from build123d import *

# Parameters (mm, degrees)
SKETCH1_W            = 12.7
SKETCH1_H            = 12.7
SKETCH1_R            = 1.25
BOSS_EXTRUDE1_DEPTH  = 3.175
SKETCH2_R            = 0.75
BOSS_EXTRUDE2_DEPTH  = 1.5
SKETCH3_R            = 0.75
CUT_EXTRUDE1_DEPTH   = 1.5
SKETCH4_W            = 12.7
SKETCH4_H            = 1
CUT_EXTRUDE2_DEPTH   = 1.75
SKETCH5_W            = 7
SKETCH5_H            = 1
CUT_EXTRUDE3_DEPTH   = 0.75
FILLET1_R            = 0.25
FILLET2_R            = 0.5
FILLET1_OF_MIRROR3_R = 0.25


with BuildPart() as part:
    # Sketch1 → Boss-Extrude1 (new body)
    with BuildSketch(Plane(origin=(0, 0, 0), x_dir=(1, 0, 0), z_dir=(0, 1, 0))):
        with Locations((-6.35, 6.35)):
            Rectangle(SKETCH1_W, SKETCH1_H)
        with Locations((-2.5, 6.35)):
            Circle(SKETCH1_R, mode=Mode.SUBTRACT)
        with Locations((-10.2, 6.35)):
            Circle(SKETCH1_R, mode=Mode.SUBTRACT)
    extrude(amount=BOSS_EXTRUDE1_DEPTH)

    # Sketch2 → Boss-Extrude2 (add)
    with BuildSketch(Plane(origin=(0, 3.175, 0), x_dir=(1, 0, 0), z_dir=(0, 1, 0))):
        with Locations((-11.2, 11.2)):
            Circle(SKETCH2_R)
    boss_extrude2 = extrude(amount=BOSS_EXTRUDE2_DEPTH)

    # Sketch3 → Cut-Extrude1 (cut)
    with BuildSketch(Plane(origin=(0, 3.175, 0), x_dir=(1, 0, 0), z_dir=(0, 1, 0))):
        with Locations((-1.5, 11.2)):
            Circle(SKETCH3_R)
    cut_extrude1 = extrude(amount=-CUT_EXTRUDE1_DEPTH, mode=Mode.SUBTRACT)

    # Mirror1: Boss-Extrude2 across plane
    add(boss_extrude2.mirror(Plane(origin=(-6.35, 0, -6.35), x_dir=(-0.707106781, 0, 0.707106781), z_dir=(-0.707106781, 0, -0.707106781))))

    # Mirror2: Cut-Extrude1 across plane
    add(cut_extrude1.mirror(Plane(origin=(0, 0, 0), x_dir=(0.707106781, 0, 0.707106781), z_dir=(-0.707106781, 0, 0.707106781))), mode=Mode.SUBTRACT)

    # Sketch4 → Cut-Extrude2 (cut)
    with BuildSketch(Plane(origin=(0, 3.175, 0), x_dir=(1, 0, 0), z_dir=(0, 1, 0))):
        with Locations((-6.35, 9.2)):
            Rectangle(SKETCH4_W, SKETCH4_H)
    cut_extrude2 = extrude(amount=-CUT_EXTRUDE2_DEPTH, mode=Mode.SUBTRACT)

    # Sketch5 → Cut-Extrude3 (cut)
    with BuildSketch(Plane(origin=(0, 1.425, 0), x_dir=(1, 0, 0), z_dir=(0, 1, 0))):
        with Locations((-6.35, 9.2)):
            Rectangle(SKETCH5_W, SKETCH5_H)
    cut_extrude3 = extrude(amount=-CUT_EXTRUDE3_DEPTH, mode=Mode.SUBTRACT)

    # Fillet1
    fillet1_edges = [part.edges().sort_by_distance(p)[0] for p in [
        (-9.85, 0.675, -9.2),
        (-2.85, 0.675, -9.2),
        (-9.85, 1.425, -9.2),
        (-2.85, 1.425, -9.2),
    ]]
    fillet(fillet1_edges, radius=FILLET1_R)

    # Fillet2
    fillet2_edges = [part.edges().sort_by_distance(p)[0] for p in [
        (0, 1.5875, 0),
        (-12.7, 1.5875, 0),
        (-12.7, 1.5875, -12.7),
        (0, 1.5875, -12.7),
    ]]
    fillet(fillet2_edges, radius=FILLET2_R)

    # Mirror3: Cut-Extrude2, Cut-Extrude3 across plane
    add(cut_extrude2.mirror(Plane(origin=(0, 0, -6.35), x_dir=(1, 0, 0), z_dir=(0, 0, -1))), mode=Mode.SUBTRACT)
    add(cut_extrude3.mirror(Plane(origin=(0, 0, -6.35), x_dir=(1, 0, 0), z_dir=(0, 0, -1))), mode=Mode.SUBTRACT)

    # Fillet1 of Mirror3
    fillet1_of_mirror3_edges = [part.edges().sort_by_distance(p)[0] for p in [
        (-9.85, 0.675, -3.5),
        (-2.85, 0.675, -3.5),
        (-9.85, 1.425, -3.5),
        (-2.85, 1.425, -3.5),
    ]]
    fillet(fillet1_of_mirror3_edges, radius=FILLET1_OF_MIRROR3_R)


solid = part.part
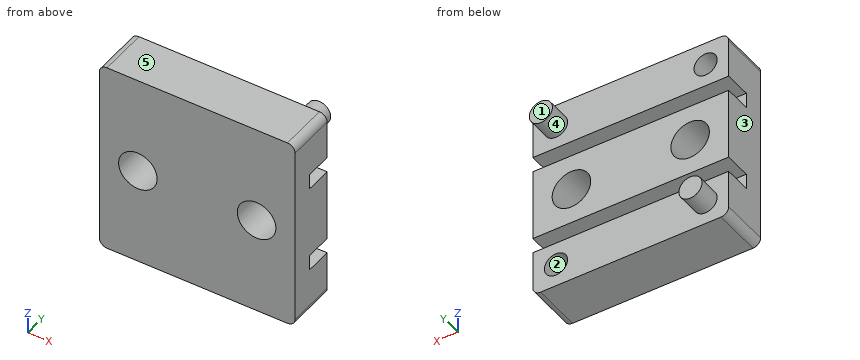
Read the model definition and answer for the solid it produces. Units are mm, in the model's axes. Face numbers are marked on the shaded views. A direction names the side the tool comes from. Give positions to 0.01 mm unless a question says otherwise; leave off trailing zeros. Write each loop counter-clockwise with the first axis right and the second up, starting at its lowest first coordinate (ties: lowest second). Pieces come first, ordered by that corner, then holes. Notation, with made-up numbers: M -11.5,31 L 33.5,31 A8 ccw 33.5,40 Z; hole C 71,32 d10. An arc over 180 degrees is marked long. One line per item, written item: value. Start each with the question number.
(1) A flat-ended cylindrical pin translates along its axis: pin 1 Ø1.6 at (x, z) = (-11, -1.5) entering from +Y (3 decimals). Find the tip coordinate at first contact, or state that the pin passes through.
(2) A tool of negligible diameter and unlimited length cuts with its end or side. For the marked faces 4 and 5, from which of +Z, -Z, +X, -X, +Y, -Y can it reach the whole face along a straight path? Write none if from no direction.
(3) Find section A-A (y = 3). Determine the outline of the cut face in (x, z), plus the area to 3 significant figures.
(4) Find section D-D (y = 3.85). Determine the outline of the cut face in (x, z).
(5) Determine the mould class of the marked faces 1, 2 and 3 for opening direction X: pulls with the +X half, pulls with the -X half, needs draft (parallel to the pull), parting line crosses it, or undercut.
(6) Find section C-C (z = -6.35). Determine the outline of the cut face in (x, y) (3 decimals).
(7) Find the intervals of material crossed by line 1 (X direction, y = 1.1, z = -6.35); line 2 (Z direction, x = -8.5, y = 1.35); line 3 (Z direction, x = -10.2, y = 2.35), in increasing order.
(8) Find section B-B (x = -11.2). Determine the outline of the cut face in (y, z) (3 decimals).
Results below:
1. pin 1: stops at y = 3.175
2. face 4: +Y
2. face 5: +Z, +X, -X, +Y, -Y
3. outline: M -12.7,-12.2 A0.5 ccw -12.2,-12.7 L -0.5,-12.7 A0.5 ccw 0,-12.2 L 0,-9.7 L -12.7,-9.7 Z; M -12.7,-8.7 L 0,-8.7 L 0,-4 L -12.7,-4 Z; M -12.7,-3 L 0,-3 L 0,-0.5 A0.5 ccw -0.5,0 L -12.2,0 A0.5 ccw -12.7,-0.5 Z; hole C -11.2,-1.5 d1.5; hole C -10.2,-6.35 d2.5; hole C -2.5,-6.35 d2.5; hole C -1.5,-11.2 d1.5
3. area: 122 mm^2
4. outline: C -11.2,-11.2 d1.5; C -1.5,-1.5 d1.5
5. face 1: needs draft
5. face 2: undercut
5. face 3: pulls with the -X half
6. outline: M -12.7,0 L -11.45,0 L -11.45,3.175 L -12.7,3.175 Z; M -8.95,0 L -3.75,0 L -3.75,3.175 L -8.95,3.175 Z; M -1.25,0 L 0,0 L 0,3.175 L -1.25,3.175 Z
7. line 1: x = -12.7 to -11.45, -8.95 to -3.75, -1.25 to 0
7. line 2: z = -12.7 to -9.7, -8.7 to -4, -3 to 0
7. line 3: z = -12.7 to -9.7, -8.7 to -7.6, -5.1 to -4, -3 to 0
8. outline: M 0,-12.7 L 3.175,-12.7 L 3.175,-11.95 L 4.675,-11.95 L 4.675,-10.45 L 3.175,-10.45 L 3.175,-9.7 L 1.425,-9.7 L 1.425,-8.7 L 3.175,-8.7 L 3.175,-7.1 L 0,-7.1 Z; M 0,-5.6 L 3.175,-5.6 L 3.175,-4 L 1.425,-4 L 1.425,-3 L 3.175,-3 L 3.175,-2.25 L 1.675,-2.25 L 1.675,-0.75 L 3.175,-0.75 L 3.175,0 L 0,0 Z
